from build123d import *

# Parameters (mm, degrees)
SKETCH2_W                = 300
SKETCH2_H                = 240
BOSS_EXTRUDE1_DEPTH      = 5
SKETCH3_R                = 1.5
CUT_EXTRUDE1_DEPTH       = 193.158788506
MIRROR2_COPY_1_SKETCH_R  = 1.5
MIRROR2_COPY_1_DEPTH     = 193.158788506
SKETCH23_W               = 65
SKETCH23_H               = 14
CUT_EXTRUDE16_DEPTH      = 193.158788506
SKETCH31_W               = 60
SKETCH31_H               = 14
CUT_EXTRUDE17_DEPTH      = 10
SKETCH45_R               = 1.5
CUT_EXTRUDE29_DEPTH      = 193.158788506
SKETCH47_R               = 1.5
CUT_EXTRUDE30_DEPTH      = 193.158788506
SKETCH48_R               = 1.5
CUT_EXTRUDE31_DEPTH      = 193.158788506
SKETCH35_R               = 1.5
CUT_EXTRUDE32_DEPTH      = 193.158788506
SKETCH9_R                = 1.5
CUT_EXTRUDE33_DEPTH      = 193.158788506
SKETCH52_R               = 1.5
CUT_EXTRUDE34_DEPTH      = 193.158788506
SKETCH10_R               = 1.5
SKETCH10_W               = 6
SKETCH10_H               = 10
CUT_EXTRUDE6_DEPTH       = 193.158788506
MIRROR13_COPY_1_SKETCH_R = 1.5
MIRROR13_COPY_1_SKETCH_W = 6
MIRROR13_COPY_1_SKETCH_H = 10
MIRROR13_COPY_1_DEPTH    = 193.158788506
SKETCH55_R               = 1.5
CUT_EXTRUDE35_DEPTH      = 193.158788506
MIRROR25_COPY_1_SKETCH_R = 1.5
MIRROR25_COPY_1_DEPTH    = 193.158788506
SKETCH59_W               = 3.430821158
SKETCH59_H               = 14
CUT_EXTRUDE37_DEPTH      = 193.158788506
SKETCH60_R               = 6.38
CUT_EXTRUDE38_DEPTH      = 193.158788506


with BuildPart() as part:
    # Sketch2 → Boss-Extrude1 (new body)
    with BuildSketch(Plane(origin=(0, 0, 0), x_dir=(1, 0, 0), z_dir=(0, 1, 0))):
        Rectangle(SKETCH2_W, SKETCH2_H)
    extrude(amount=BOSS_EXTRUDE1_DEPTH)

    # Sketch3 → Cut-Extrude1 (cut, through all)
    with BuildSketch(Plane(origin=(0, 5, 0), x_dir=(1, 0, 0), z_dir=(0, 1, 0))):
        with Locations(Location((142.5, 112.5, 0), (0, 0, 270))):
            Circle(SKETCH3_R)
    cut_extrude1 = extrude(amount=-CUT_EXTRUDE1_DEPTH, mode=Mode.SUBTRACT)

    # Mirror1: Cut-Extrude1 across plane
    add(cut_extrude1.mirror(Plane(origin=(0, 0, 0), x_dir=(0, 0, 1), z_dir=(1, 0, 0))), mode=Mode.SUBTRACT)

    # Mirror2: Cut-Extrude1 across plane
    add(cut_extrude1.mirror(Plane.XY), mode=Mode.SUBTRACT)

    # Mirror2 copy 1 sketch → Mirror2 copy 1 (cut, through all)
    with BuildSketch(Plane(origin=(0, 5, 0), x_dir=(-1, 0, 0), z_dir=(0, 1, 0))):
        with Locations(Location((142.5, 112.5, 0), (0, 0, 270))):
            Circle(MIRROR2_COPY_1_SKETCH_R)
    extrude(amount=-MIRROR2_COPY_1_DEPTH, mode=Mode.SUBTRACT)

    # Sketch23 → Cut-Extrude16 (cut, through all)
    with BuildSketch(Plane(origin=(0, 5, 0), x_dir=(1, 0, 0), z_dir=(0, 1, 0))):
        with Locations((-27.5, -113)):
            Rectangle(SKETCH23_W, SKETCH23_H)
    cut_extrude16 = extrude(amount=-CUT_EXTRUDE16_DEPTH, mode=Mode.SUBTRACT)

    # Sketch31 → Cut-Extrude17 (cut)
    with BuildSketch(Plane(origin=(0, 5, 0), x_dir=(1, 0, 0), z_dir=(0, 1, 0))):
        with Locations((85, -113)):
            Rectangle(SKETCH31_W, SKETCH31_H)
    cut_extrude17 = extrude(amount=-CUT_EXTRUDE17_DEPTH, mode=Mode.SUBTRACT)

    # Mirror14: Cut-Extrude16 across plane
    add(cut_extrude16.mirror(Plane.XY), mode=Mode.SUBTRACT)

    # Sketch45 → Cut-Extrude29 (cut, through all)
    with BuildSketch(Plane(origin=(0, 5, 0), x_dir=(1, 0, 0), z_dir=(0, 1, 0))):
        with Locations(Location((-44.788992857, 42.236040749, 0), (0, 0, 270))):
            Circle(SKETCH45_R)
    extrude(amount=-CUT_EXTRUDE29_DEPTH, mode=Mode.SUBTRACT)

    # Sketch47 → Cut-Extrude30 (cut, through all)
    with BuildSketch(Plane(origin=(0, 5, 0), x_dir=(1, 0, 0), z_dir=(0, 1, 0))):
        with Locations(Location((60.211007143, -45.763959251, 0), (0, 0, 270))):
            Circle(SKETCH47_R)
    extrude(amount=-CUT_EXTRUDE30_DEPTH, mode=Mode.SUBTRACT)

    # Sketch48 → Cut-Extrude31 (cut, through all)
    with BuildSketch(Plane(origin=(0, 5, 0), x_dir=(1, 0, 0), z_dir=(0, 1, 0))):
        with Locations(Location((60.211007143, 42.236040749, 0), (0, 0, 270))):
            Circle(SKETCH48_R)
    extrude(amount=-CUT_EXTRUDE31_DEPTH, mode=Mode.SUBTRACT)

    # Sketch35 → Cut-Extrude32 (cut, through all)
    with BuildSketch(Plane(origin=(0, 5, 0), x_dir=(1, 0, 0), z_dir=(0, 1, 0))):
        with Locations(Location((-44.788992857, -45.763959251, 0), (0, 0, 270))):
            Circle(SKETCH35_R)
    extrude(amount=-CUT_EXTRUDE32_DEPTH, mode=Mode.SUBTRACT)

    # Sketch9 → Cut-Extrude33 (cut, through all)
    with BuildSketch(Plane(origin=(0, 0, 0), x_dir=(-1, 0, 0), z_dir=(0, -1, 0))):
        with Locations(Location((28, -39.25, 0), (0, 0, 90))):
            Circle(SKETCH9_R)
    extrude(amount=-CUT_EXTRUDE33_DEPTH, mode=Mode.SUBTRACT)

    # Sketch52 → Cut-Extrude34 (cut, through all)
    with BuildSketch(Plane(origin=(0, 5, 0), x_dir=(1, 0, 0), z_dir=(0, 1, 0))):
        with Locations(Location((-28, 16.75, 0), (0, 0, 270))):
            Circle(SKETCH52_R)
        with Locations(Location((50.5, 16.75, 0), (0, 0, 270))):
            Circle(SKETCH52_R)
        with Locations(Location((50.5, -39.25, 0), (0, 0, 270))):
            Circle(SKETCH52_R)
    extrude(amount=-CUT_EXTRUDE34_DEPTH, mode=Mode.SUBTRACT)

    # Mirror20: Cut-Extrude17 across plane
    add(cut_extrude17.mirror(Plane.XY), mode=Mode.SUBTRACT)

    # Sketch10 → Cut-Extrude6 (cut, through all)
    with BuildSketch(Plane(origin=(0, 5, 0), x_dir=(1, 0, 0), z_dir=(0, 1, 0))):
        with Locations(Location((-122.5, -67, 0), (0, 0, 270))):
            Circle(SKETCH10_R)
        with Locations((-144.3, -67)):
            Rectangle(SKETCH10_W, SKETCH10_H)
    cut_extrude6 = extrude(amount=-CUT_EXTRUDE6_DEPTH, mode=Mode.SUBTRACT)

    # Mirror12: Cut-Extrude6 across plane
    add(cut_extrude6.mirror(Plane.XY), mode=Mode.SUBTRACT)

    # Mirror13: Cut-Extrude6 across plane
    add(cut_extrude6.mirror(Plane(origin=(0, 0, 0), x_dir=(0, 0, 1), z_dir=(1, 0, 0))), mode=Mode.SUBTRACT)

    # Mirror13 copy 1 sketch → Mirror13 copy 1 (cut, through all)
    with BuildSketch(Plane(origin=(0, 5, 0), x_dir=(-1, 0, 0), z_dir=(0, 1, 0))):
        with Locations(Location((-122.5, -67, 0), (0, 0, 270))):
            Circle(MIRROR13_COPY_1_SKETCH_R)
        with Locations((-144.3, -67)):
            Rectangle(MIRROR13_COPY_1_SKETCH_W, MIRROR13_COPY_1_SKETCH_H)
    extrude(amount=-MIRROR13_COPY_1_DEPTH, mode=Mode.SUBTRACT)

    # Sketch55 → Cut-Extrude35 (cut, through all)
    with BuildSketch(Plane(origin=(0, 5, 0), x_dir=(1, 0, 0), z_dir=(0, 1, 0))):
        with Locations(Location((-31.5, -95, 0), (0, 0, 270))):
            Circle(SKETCH55_R)
        with Locations(Location((-15.5, -80.653573709, 0), (0, 0, 270))):
            Circle(SKETCH55_R)
        with Locations(Location((-15.5, -94.653573709, 0), (0, 0, 270))):
            Circle(SKETCH55_R)
        with Locations(Location((-31.5, -80.653573709, 0), (0, 0, 270))):
            Circle(SKETCH55_R)
    cut_extrude35 = extrude(amount=-CUT_EXTRUDE35_DEPTH, mode=Mode.SUBTRACT)

    # Mirror24: Cut-Extrude35 across plane
    add(cut_extrude35.mirror(Plane(origin=(30, 0, 0), x_dir=(0, 0, 1), z_dir=(1, 0, 0))), mode=Mode.SUBTRACT)

    # Mirror25: Cut-Extrude35 across plane
    add(cut_extrude35.mirror(Plane.XY), mode=Mode.SUBTRACT)

    # Mirror25 copy 1 sketch → Mirror25 copy 1 (cut, through all)
    with BuildSketch(Plane(origin=(60, 5, 0), x_dir=(-1, 0, 0), z_dir=(0, 1, 0))):
        with Locations(Location((-31.5, -95, 0), (0, 0, 270))):
            Circle(MIRROR25_COPY_1_SKETCH_R)
        with Locations(Location((-15.5, -80.653573709, 0), (0, 0, 270))):
            Circle(MIRROR25_COPY_1_SKETCH_R)
        with Locations(Location((-15.5, -94.653573709, 0), (0, 0, 270))):
            Circle(MIRROR25_COPY_1_SKETCH_R)
        with Locations(Location((-31.5, -80.653573709, 0), (0, 0, 270))):
            Circle(MIRROR25_COPY_1_SKETCH_R)
    extrude(amount=-MIRROR25_COPY_1_DEPTH, mode=Mode.SUBTRACT)

    # Sketch59 → Cut-Extrude37 (cut, through all)
    with BuildSketch(Plane(origin=(0, 5, 0), x_dir=(1, 0, 0), z_dir=(0, 1, 0))):
        with Locations((53.284589421, -113)):
            Rectangle(SKETCH59_W, SKETCH59_H)
    extrude(amount=-CUT_EXTRUDE37_DEPTH, mode=Mode.SUBTRACT)

    # Sketch60 → Cut-Extrude38 (cut, through all)
    with BuildSketch(Plane(origin=(0, 5, 0), x_dir=(1, 0, 0), z_dir=(0, 1, 0))):
        with Locations(Location((-90.412183362, 0, 0), (0, 0, 270))):
            Circle(SKETCH60_R)
    extrude(amount=-CUT_EXTRUDE38_DEPTH, mode=Mode.SUBTRACT)


solid = part.part
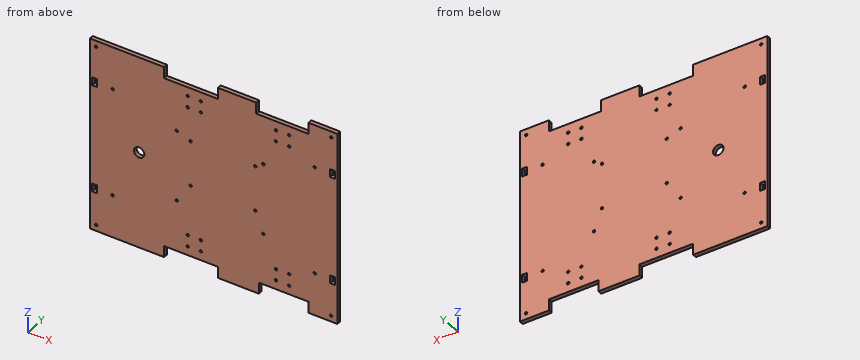
Could you check a few things on this model? Use its own coordinates, in mm. Round coordinates to 2 decimals unless told otherwise and drop trailing zeros. Order: outer loops, then holes, each group sorted by start corner. A loop starts at its lowest first (then second) coordinate and runs counter-clockwise, first axis right, second up.
(1) Imagine slicing it at A-A (x = -51.5). Write out the boundary of the cut face in (y, z).
Response values:
outline: (0, -106) - (5, -106) - (5, 106) - (0, 106) - close
(2) Please list where these lines run through material, in increasing order: line 1 along Z through (x, y) = (75.5, 2.85); line 2 along X through (y, z) = (3.8, -112.5); line 3 along X through (y, z) = (2.35, 95).
Response values:
line 1: z = -106 to -96.15, -93.15 to -82.15, -79.15 to 79.15, 82.15 to 93.15, 96.15 to 106
line 2: x = -150 to -144, -141 to -60, 5 to 55, 115 to 141, 144 to 150
line 3: x = -150 to -33, -30 to -16.96, -14.04 to 74.04, 76.96 to 90, 93 to 150
(3) I'm going to push flat-ended pins straight in: pin 1 (5 mm diameter, centred on x = -15.5, z = 94.65, fed in from -Y); pin 2 (2.5 mm diameter, centred on x = 91.5, z = 80.65, fed in from +Y); pin 3 (2.5 mm diameter, centred on x = 91, y = 2.5, fed in from +Z); pin 4 (1.5 mm diameter, centred on x = 64.5, y = 2, fed in from -Z). Where does each tip first touch, or does it pass through?
Response values:
pin 1: stops at y = 0
pin 2: passes through
pin 3: stops at z = 106
pin 4: stops at z = -106
(4) Imagine slicing it at B-B (y = 2.85). Count the separate pieces of the cut face and the enclosed holes in it, plus the area to 3 significant figures.
Response values:
separate pieces: 1
enclosed holes: 37
area: 67,900 mm2
